Read the model definition and answer for the solid it produces. Units are mm, in the model's axes. Coordinates: 2 decimals unless noted, no trailing zeros. Order: outer loops, then holes, each group sorted by start corner. A loop starts at its lowest first (then second) coordinate and runs counter-clockwise, first axis right, second up. Notation, with made-up numbers: (35.25, 77.5) -> (48.25, 77.5) arc R27 cw to (48.25, 96.5) -> close; hole circle Ø9 at (36, 22). An arc over 180 degrees is marked (long way). Answer as a JSON object with one key per item and string values. Group by question number.
1) Section B-B on z = 12 is taken. Determine the outline of the cut face in (x, y).
2) Section C-C on y = 0 is taken. Determine the outline of the cut face in (x, z), and give its area (3 significant figures).
3) Section A-A on x = 0 is taken. Determine the outline of the cut face in (y, z).
4) Section D-D on x = -30 is taken. Determine the outline of the cut face in (y, z).
5) Consider L1, parallel to Y at x = 0, z = 0.8; L2, parallel to X at y = 18, z = 1; L3, parallel to Z at x = -12.5, y = 6.5. Determine where each line is inside the solid, lowest interval first.
6) Given pin 1 (4 mm diameter, centred on x = 0, y = 23.01, fed in from -Z); pin 2 (12 mm diameter, centred on x = -27, z = 3, fed in from +Y); pin 3 (6 mm diameter, centred on x = 4, z = 12.5, fed in from +Y); pin 4 (4 mm diameter, centred on x = -19.5, y = 4, fed in from -Z), each flat-ended and moving along its own axis, determine where each tip first touches the part or whether it passes through.
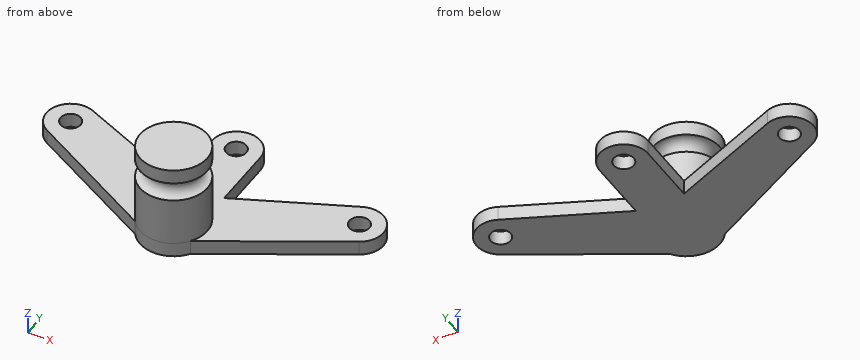
from build123d import *

# Parameters (mm, degrees)
TORUS001_R        = 2
SKETCH003_R       = 2.1
PAD003_DEPTH      = 3
CYLINDER005_R     = 7
CYLINDER005_DEPTH = 20


with BuildPart() as torus001:
    # Torus001 → Torus001 (revolve)
    with BuildSketch(Plane(origin=(0, 0, 15), x_dir=(1, 0, 0), z_dir=(0, -1, 0))):
        with Locations((7, 0)):
            Circle(TORUS001_R)
    revolve(axis=Axis((0, 0, 15), (0, 0, 1)))


with BuildPart() as base_body001:
    # Sketch003 → Pad003 (new body)
    with BuildSketch(Plane.XY):
        with BuildLine():
            Line((-32.430713, 10.8347), (-5.732093, -4.017849))
            ThreePointArc((-5.732093, -4.017849), (0, -7), (5.732093, -4.017849))
            Line((5.732093, -4.017849), (32.430713, 10.8347))
            ThreePointArc((32.430713, 10.8347), (34.479244, 17.425892), (27.992075, 19.783207))
            Line((5, 9.701256), (27.992075, 19.783207))
            Line((5, 23.014347), (5, 9.701256))
            ThreePointArc((5, 23.014347), (0, 28.014347), (-5, 23.014347))
            Line((-5, 9.701256), (-5, 23.014347))
            Line((-27.992075, 19.783207), (-5, 9.701256))
            ThreePointArc((-27.992075, 19.783207), (-34.479244, 17.425892), (-32.430713, 10.8347))
        make_face()
        with Locations((-30, 15.204098)):
            Circle(SKETCH003_R, mode=Mode.SUBTRACT)
        with Locations((30, 15.204098)):
            Circle(SKETCH003_R, mode=Mode.SUBTRACT)
        with Locations((0, 23.014347)):
            Circle(SKETCH003_R, mode=Mode.SUBTRACT)
    extrude(amount=PAD003_DEPTH)


with BuildPart() as base_cut_for_big_metal_plate:
    # Cylinder005 → Cylinder005 (new body)
    with BuildSketch(Plane.XY):
        Circle(CYLINDER005_R)
    extrude(amount=CYLINDER005_DEPTH)

    # Fusion005: union base body001
    add(base_body001.part)

    # Cut003004: cut Torus001
    add(torus001.part, mode=Mode.SUBTRACT)


solid = base_cut_for_big_metal_plate.part
Worked answers:
{
 "1": {"outline": "circle Ø14 at (0, 0)"},
 "2": {"outline": "(-12.95, 0) -> (12.95, 0) -> (12.95, 3) -> (7, 3) -> (7, 13) arc R2 cw to (7, 17) -> (7, 20) -> (-7, 20) -> (-7, 17) arc R2 cw to (-7, 13) -> (-7, 3) -> (-12.95, 3) -> close", "area": "303 mm²"},
 "3": {"outline": "(-7, 0) -> (20.91, 0) -> (20.91, 3) -> (7, 3) -> (7, 13) arc R2 cw to (7, 17) -> (7, 20) -> (-7, 20) -> (-7, 17) arc R2 cw to (-7, 13) -> close; (25.11, 0) -> (28.01, 0) -> (28.01, 3) -> (25.11, 3) -> close"},
 "4": {"outline": "(9.48, 0) -> (13.1, 0) -> (13.1, 3) -> (9.48, 3) -> close; (17.3, 0) -> (20.2, 0) -> (20.2, 3) -> (17.3, 3) -> close"},
 "5": {"L1": "y = -7 to 20.91, 25.11 to 28.01", "L2": "x = -34.15 to -23.93, -5 to 5, 23.93 to 34.15", "L3": "z = 0 to 3"},
 "6": {"pin 1": "passes through", "pin 2": "stops at y = 20.2", "pin 3": "stops at y = 6.93", "pin 4": "stops at z = 0"}
}
